```python
from build123d import *

# Parameters (mm, degrees)
SKETCH_1_R          = 1
EXTRUDE_1_DEPTH     = 1.6
SKETCH_2_R          = 1
CUT_EXTRUDE_1_DEPTH = 1.6
EXTRUDE_START       = 1.6
SKETCH_4_W          = 18.99
SKETCH_4_H          = 15.2
EXTRUDE_2_DEPTH     = 9.2
CUT_EXTRUDE_START   = 42.7
CUT_EXTRUDE_2_DEPTH = 15.2
SKETCH_6_W          = 15.54
SKETCH_6_H          = 1.6
CUT_EXTRUDE_3_DEPTH = 9
SKETCH_7_W          = 31.69
SKETCH_7_H          = 15.2
EXTRUDE_3_DEPTH     = 9.2
CUT_EXTRUDE_START_2 = -37.7
SKETCH_9_W          = 28.24
SKETCH_9_H          = 1.6
CUT_EXTRUDE_5_DEPTH = 9
CUT_EXTRUDE_6_DEPTH = 15.2


with BuildPart() as part:
    # 草图1 → 凸台-拉伸1 (new body)
    with BuildSketch(Plane.XY):
        with BuildLine():
            Line((-13, 32.5), (13, 32.5))
            ThreePointArc((13, 32.5), (14.414213562, 31.914213562), (15, 30.5))
            Line((15, 30.5), (15, -25.5))
            ThreePointArc((15, -25.5), (14.414213562, -26.914213562), (13, -27.5))
            Line((13, -27.5), (-13, -27.5))
            ThreePointArc((-13, -27.5), (-14.414213562, -26.914213562), (-15, -25.5))
            Line((-15, -25.5), (-15, 30.5))
            ThreePointArc((-15, 30.5), (-14.414213562, 31.914213562), (-13, 32.5))
        make_face()
        with Locations((-13, 30.5)):
            Circle(SKETCH_1_R, mode=Mode.SUBTRACT)
        with Locations((13, 30.5)):
            Circle(SKETCH_1_R, mode=Mode.SUBTRACT)
    extrude(amount=EXTRUDE_1_DEPTH)

    # 草图2 → 切除-拉伸1 (cut)
    with BuildSketch(Plane.XY):
        with Locations((-13, -5.5)):
            Circle(SKETCH_2_R)
        with Locations((13, -5.5)):
            Circle(SKETCH_2_R)
    extrude(amount=CUT_EXTRUDE_1_DEPTH, mode=Mode.SUBTRACT)

    # 草图4 → 凸台-拉伸2 (add)
    with BuildSketch(Plane.XY.offset(EXTRUDE_START)):
        with Locations((0, 35.1)):
            Rectangle(SKETCH_4_W, SKETCH_4_H)
    extrude(amount=EXTRUDE_2_DEPTH)

    # 草图5 → 切除-拉伸2 (cut)
    with BuildSketch(Plane(origin=(0, 0, 0), x_dir=(1, 0, 0), z_dir=(0, 1, 0)).offset(CUT_EXTRUDE_START)):
        Polygon((-9.495, -10.8), (-8.495, -10.8), (-9.495, -9.8), align=None)
        Polygon((9.495, -10.8), (8.495, -10.8), (9.495, -9.8), align=None)
        Polygon((9.495, -1.6), (9.495, -2.6), (8.495, -1.6), align=None)
        Polygon((-9.495, -1.6), (-8.495, -1.6), (-9.495, -2.6), align=None)
    extrude(amount=-CUT_EXTRUDE_2_DEPTH, mode=Mode.SUBTRACT)

    # 草图6 → 切除-拉伸3 (cut)
    with BuildSketch(Plane(origin=(0, 0, 0), x_dir=(1, 0, 0), z_dir=(0, 1, 0)).offset(CUT_EXTRUDE_START)):
        with Locations((0, -6.2)):
            Rectangle(SKETCH_6_W, SKETCH_6_H)
    extrude(amount=-CUT_EXTRUDE_3_DEPTH, mode=Mode.SUBTRACT)

    # 草图7 → 凸台-拉伸3 (add)
    with BuildSketch(Plane.XY.offset(EXTRUDE_START)):
        with Locations((0, -30.1)):
            Rectangle(SKETCH_7_W, SKETCH_7_H)
    extrude(amount=EXTRUDE_3_DEPTH)

    # 草图9 → 切除-拉伸5 (cut)
    with BuildSketch(Plane(origin=(0, 0, 0), x_dir=(1, 0, 0), z_dir=(0, 1, 0)).offset(CUT_EXTRUDE_START_2)):
        with Locations((0, -6.2)):
            Rectangle(SKETCH_9_W, SKETCH_9_H)
    extrude(amount=CUT_EXTRUDE_5_DEPTH, mode=Mode.SUBTRACT)

    # 草图10 → 切除-拉伸6 (cut)
    with BuildSketch(Plane(origin=(0, 0, 0), x_dir=(1, 0, 0), z_dir=(0, 1, 0)).offset(CUT_EXTRUDE_START_2)):
        Polygon((15.845, -10.8), (14.845, -10.8), (15.845, -9.8), align=None)
        Polygon((-15.845, -10.8), (-14.845, -10.8), (-15.845, -9.8), align=None)
        Polygon((-15.845, -2.6), (-14.845, -1.6), (-15.845, -1.6), align=None)
        Polygon((15.845, -2.6), (14.845, -1.6), (15.845, -1.6), align=None)
    extrude(amount=CUT_EXTRUDE_6_DEPTH, mode=Mode.SUBTRACT)


solid = part.part
```
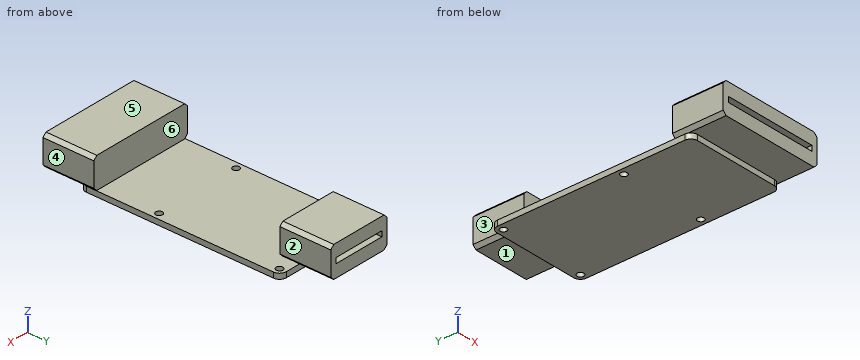
For this review, take the finished solid that the model builds, in its own axes (mm). Face numbers are marked on the shaded views. A direction names the side the tool comes from. Round coordinates to 2 decimals unless told otherwise and drop trailing zeros. Loops run counter-clockwise (first coordinate to the right, second up) from the corner with the lowest first, then second, coordinate; pieces in that order, holes last.
(1) We need section C-C (x = -4). Give the boundary of the cut face in (y, z), plus the area to 3 significant figures.
Returned:
outline: (-37.7, 1.6) - (-27.5, 1.6) - (-27.5, 0) - (32.5, 0) - (32.5, 1.6) - (42.7, 1.6) - (42.7, 5.4) - (33.7, 5.4) - (33.7, 7) - (42.7, 7) - (42.7, 10.8) - (27.5, 10.8) - (27.5, 1.6) - (-22.5, 1.6) - (-22.5, 10.8) - (-37.7, 10.8) - (-37.7, 7) - (-28.7, 7) - (-28.7, 5.4) - (-37.7, 5.4) - close
area: 347 mm2
(2) Clearance check with flat-ended pins moving along their axes: P1, Ø5, axis at x = 3, y = 36.5, coming from the -Z side; P2, Ø9, axis at x = 4.5, y = 7.5, coming from the +Z side; P3, Ø1.8, axis at y = 16, z = 0.5, coming from the +X side. State where each tip first meets the part, or that it passes through.
Returned:
P1: stops at z = 1.6
P2: stops at z = 1.6
P3: stops at x = 15
(3) Wall thickness on line 1 along Y through (x, z) = (-13, 1.25); line 2 along Z through (x, y) = (0, -31.5); line 3 along Y through (x, z) = (7, 9.25): over which ranges is each line inside the solid? List them lowest first.
Returned:
line 1: y = -27.5 to -6.5, -4.5 to 29.5, 31.5 to 32.5
line 2: z = 1.6 to 5.4, 7 to 10.8
line 3: y = -37.7 to -22.5, 27.5 to 42.7
(4) Mouldability with a two-part tool opening along Y and no side actions: class the marked faces 5 and 6 as released by +Y, released by -Y, zero draft, split by the parting line, or undercut.
Returned:
face 5: zero draft
face 6: undercut
(5) Tool access review of the marked faces 1, 2, 3 and 4: name each direction out of +Z, -Z, +X, -X, +Y, -Y from which nothing blocks a thin tool from reaching the whole face with its end or side.
Returned:
face 1: -Z, +X, -X, +Y
face 2: +Z, +X, +Y
face 3: +Z, -X, +Y
face 4: +Z, -Z, +X, +Y, -Y
(6) We need section A-A (y = -5.5). Give the boundary of the cut face in (x, z).
Returned:
outline: (-15, 0) - (-14, 0) - (-14, 1.6) - (-15, 1.6) - close; (-12, 0) - (12, 0) - (12, 1.6) - (-12, 1.6) - close; (14, 0) - (15, 0) - (15, 1.6) - (14, 1.6) - close
(7) We need section B-B (z = 8.25). Give the boundary of the cut face in (x, y) (3 decimals), plus the area to 3 significant figures.
Returned:
outline: (-15.845, -37.7) - (15.845, -37.7) - (15.845, -22.5) - (-15.845, -22.5) - close; (-9.495, 27.5) - (9.495, 27.5) - (9.495, 42.7) - (-9.495, 42.7) - close
area: 770 mm2
(8) We need section D-D (y = -18.5). Give the boundary of the cut face in (x, z).
Returned:
outline: (-15, 0) - (15, 0) - (15, 1.6) - (-15, 1.6) - close
